Check sheet for the modelled part. Datum: model origin and axes. Units: mm. A direction names the side the tool comes from. Round coordinates to 2 decimals unless told otherwise and drop trailing zeros. Write each loop counter-clockwise with the first axis right and the second up, starting at its lowest first coordinate (ties: lowest second). Pieces come first, ordered by that corner, then holes. Notation, with made-up numbers: (58.5, 86) - (89.5, 86) arc R21 ccw to (89.5, 119) - close; hole circle Ø1 at (-10.5, 10). An arc over 180 degrees is marked (long way). Use one line per item in the form item = value. Start each with the question number.
1) Section check B-B (x = -110). Record the boundary of the cut face in (y, z).
2) Scan lines: probe 1 along Y at (x, z) = (-25, -1); probe 2 along Z at (x, y) = (-61, -26); probe 3 along X at (y, z) = (-18, -1.5). Record each from-to range of solid material in increasing order.
3) Draft check along Y on faces 1 (the face through (-80.4, -60, 17.2)), 2 (the face through (-80.4, 0, 17.2)), 3 (the face through (-30, -30, -2)), 4 (the face through (-39, -30, 0)). Enter one of: +Y half, -Y half, draft (parallel to the pull), parting line (faces both ways), or undercut.
4) Section check C-C (y = -17). Record the boundary of the cut face in (x, z).
5) Set-up check for faces 5 (the face through (-80, -30, 17)), 6 (the face through (-160, -30, 31)), 7 (the face through (-123, -36, 28.534)), 8 (the face through (-120, -25, 31)): record each of +Z, -Z, +X, -X, +Y, -Y from which the full face is reachable in a straight line by a thin tool's end or side.
6) Section check A-A (y = -30). Record the boundary of the cut face in (x, z).
7) Gauge pin test, flat ends, axial feed: P1, Ø17, axis at y = -32, z = 4.5, coming from the -X side; P2, Ø6, axis at x = -25, y = -30, coming from the -Z side (3 decimals); P3, Ø4, axis at y = -25.5, z = 18.5, coming from the +X side. Record the tip position at first contact, or that the pin passes through.
8) Section check D-D (x = -24). Record the boundary of the cut face in (y, z).
from build123d import *

# Parameters (mm, degrees)
F1_DEPTH = 60
F2_R     = 5
F3_DEPTH = 50
F4_R     = 5


with BuildPart() as f1:
    # F0 (on Front) → F1 (new body)
    with BuildSketch(Plane.XZ):
        Polygon((0, -5), (0, 0), (-80, 0), (-80, 33.534), (-160, 33.534), (-160, 28.534), (-85, 28.534), (-85, -5), align=None)
    extrude(amount=F1_DEPTH)

    # F2 (on face) → F3 (cut, symmetric)
    with BuildSketch(Plane.XY):
        with Locations((-25, -30)):
            Circle(F2_R)
        with BuildLine():
            Line((-105, -25), (-135, -25))
            ThreePointArc((-135, -25), (-140, -30), (-135, -35))
            Line((-135, -35), (-105, -35))
            ThreePointArc((-105, -35), (-100, -30), (-105, -25))
        make_face()
    extrude(amount=F3_DEPTH, both=True, mode=Mode.SUBTRACT)

    # F4
    f4_edges = [f1.edges().sort_by_distance(p)[0] for p in [
        (-160, -60, 31.034),
        (-160, 0, 31.034),
        (0, -60, -2.5),
        (0, 0, -2.5),
    ]]
    fillet(f4_edges, radius=F4_R)


solid = f1.part
Results are:
q1.outline = (-60, 28.53) - (-35, 28.53) - (-35, 33.53) - (-60, 33.53) - close; (-25, 28.53) - (0, 28.53) - (0, 33.53) - (-25, 33.53) - close
q2.probe_1 = -60 to -35, -25 to 0
q2.probe_2 = -5 to 0
q2.probe_3 = -85 to 0
q3.face_1 = -Y half
q3.face_2 = +Y half
q3.face_3 = undercut
q3.face_4 = draft
q4.outline = (-160, 28.53) - (-85, 28.53) - (-85, -5) - (0, -5) - (0, 0) - (-80, 0) - (-80, 33.53) - (-160, 33.53) - close
q5.face_5 = +Z, +X, +Y, -Y
q5.face_6 = +Z, -Z, -X, +Y, -Y
q5.face_7 = -Z, -X, +Y, -Y
q5.face_8 = +Z, -Z
q6.outline = (-160, 28.53) - (-140, 28.53) - (-140, 33.53) - (-160, 33.53) - close; (-100, 28.53) - (-85, 28.53) - (-85, -5) - (-30, -5) - (-30, 0) - (-80, 0) - (-80, 33.53) - (-100, 33.53) - close; (-20, -5) - (0, -5) - (0, 0) - (-20, 0) - close
q7.P1 = -85
q7.P2 = through
q7.P3 = -80
q8.outline = (-60, -5) - (-34.9, -5) - (-34.9, 0) - (-60, 0) - close; (-25.1, -5) - (0, -5) - (0, 0) - (-25.1, 0) - close
